```python
from build123d import *

# Parameters (mm, degrees)
SKETCH1_R           = 24.5
SKETCH1_R_2         = 3.5
SKETCH1_R_3         = 4
BOSS_EXTRUDE1_DEPTH = 4.5
SKETCH2_R           = 16
CUT_EXTRUDE1_DEPTH  = 2
CHAMFER1_SIZE       = 2
CHAMFER2_SIZE       = 1


with BuildPart() as part:
    # Sketch1 → Boss-Extrude1 (new, symmetric)
    with BuildSketch(Plane.XY):
        Circle(SKETCH1_R)
        with Locations((0, 12)):
            Circle(SKETCH1_R_2, mode=Mode.SUBTRACT)
        with Locations((-12, 0)):
            Circle(SKETCH1_R_2, mode=Mode.SUBTRACT)
        with Locations((0, -12)):
            Circle(SKETCH1_R_2, mode=Mode.SUBTRACT)
        with Locations((12, 0)):
            Circle(SKETCH1_R_2, mode=Mode.SUBTRACT)
        Circle(SKETCH1_R_3, mode=Mode.SUBTRACT)
    extrude(amount=BOSS_EXTRUDE1_DEPTH, both=True)

    # Sketch2 → Cut-Extrude1 (cut)
    with BuildSketch(Plane.XY.offset(4.5)):
        Circle(SKETCH2_R)
    extrude(amount=-CUT_EXTRUDE1_DEPTH, mode=Mode.SUBTRACT)

    # Chamfer1
    chamfer1_edges = [part.edges().sort_by_distance(p)[0] for p in [
        (-16, 0, 4.5),
    ]]
    chamfer(chamfer1_edges, length=CHAMFER1_SIZE - 0.0001)  # a hair under: the kernel refuses the full size

    # Chamfer2
    chamfer2_edges = [part.edges().sort_by_distance(p)[0] for p in [
        (-24.5, 0, 4.5),
    ]]
    chamfer(chamfer2_edges, length=CHAMFER2_SIZE)


solid = part.part
```
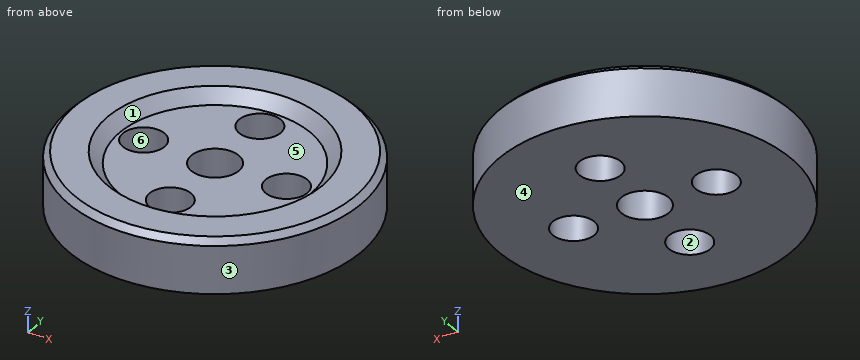
Read the model definition and answer for the solid it produces. Units are mm, in the model's axes. Face numbers are marked on the shaded views. A direction names the side the tool comes from. Give positions to 0.01 mm unless a question says otherwise; leave off trailing zeros. Loops run counter-clockwise (first coordinate to the right, second up) from the corner with the lowest first, then second, coordinate; pieces in that order, holes last.
Item 1: For the marked faces 5 and 6, determine the directions among +Z, -Z, +X, -X, +Y, -Y from which every point of the face is accessible in a straight line to the end or side of a thin tool.
Item 2: The part is cut by section A-A (x = 0). Give the number of separate pieces and of enclosed holes in the cut face, and give its area (3 significant figures).
Item 3: The mould has two halves that part along X. Classify the marked faces 1, 2, 3 and 4: released by +X, released by -X, zero draft, split by the parting line, or undercut.
Item 4: The part is cut by section C-C (z = -1). Write down the section's boundary in (x, y), and give its area (3 significant figures).
Item 5: Each of these flat-tipped pins is pushed along its axis until it touches: pin 1 Ø2 at (x, y) = (7.5, 14) entering from +Z; pin 2 Ø3 at (y, z) = (-18.5, 1) entering from +X; pin 3 Ø1 at (x, z) = (-3.5, 1) entering from +Y. Where does it stop, or does it pass through?
Item 6: Find the intervals of material crossed by line 1 along Y through (x, z) = (0, -1.25); line 2 along Z through (x, y) = (7, 6); line 3 along X through (y, z) = (-11, 0.75), in increasing order.
Taken from the geometry:
1. face 5: +Z
1. face 6: +Z, -Z
2. separate pieces: 4
2. enclosed holes: 0
2. area: 218 mm2
3. face 1: undercut
3. face 2: undercut
3. face 3: split by the parting line
3. face 4: zero draft
4. outline: circle Ø49 at (0, 0); hole circle Ø7 at (-12, 0); hole circle Ø8 at (0, 0); hole circle Ø7 at (0, -12); hole circle Ø7 at (0, 12); hole circle Ø7 at (12, 0)
4. area: 1,680 mm2
5. pin 1: stops at z = 3.38
5. pin 2: stops at x = 17.64
5. pin 3: stops at y = 24.32
6. line 1: y = -24.5 to -15.5, -8.5 to -4, 4 to 8.5, 15.5 to 24.5
6. line 2: z = -4.5 to 2.5
6. line 3: x = -21.89 to -3.35, 3.35 to 21.89
